For this review, take the finished solid that the model builds, in its own axes (mm). A direction names the side the tool comes from. Give positions to 0.01 mm unless a question says otherwise; leave off trailing zeros. Write each loop counter-clockwise with the first axis right and the second up, starting at its lowest first coordinate (ties: lowest second). Pieces come first, ordered by that corner, then holes. Notation, with made-up numbers: M 62.5,21 L 84.5,21 A34 cw 84.5,51 Z; hole C 35,13.5 d4. An arc over 180 degrees is marked long. One line per item, written item: value. Start each with the question number.
Item 1: Consider section B-B, the plane y = 35.5. Give the number of separate pieces and of enclosed holes in the cut face, and give its area (3 significant figures).
Item 2: Tool access review of faces 4 (the face through (-21.958, 49.233, 61.115)), 5 (the face through (-18.739, 41, 58)), 6 (the face through (-8.96, 43, 63)), 7 (the face through (53.62, 34.34, 48.98)): name each direction out of +Z, -Z, +X, -X, +Y, -Y from which nothing blocks a thin tool from reaching the whole face with its end or side.
Item 3: Consider section D-D, the plane y = 47. Write out the cut boundary in (x, z).
Item 4: Consider section C-C, the plane z = 41. Write out the cut boundary in (x, y).
Item 5: Clearance check with flat-ended pins moving along their axes: pin 1 Ø4 at (x, z) = (55.25, 77) entering from +Y; pin 2 Ø4 at (x, z) = (51, 32) entering from +Y; pin 3 Ø4 at (x, z) = (55.25, 49.05) entering from -Y. State where each tip first meets the part, or that it passes through.
Item 6: Mouldability with a two-part tool opening along Y and no side actions: class faces 1 (the face through (20, 47, 29.962)), 2 (the face through (-13.918, 52.936, 53.683)), 3 (the face through (57, 39.124, 78)) as released by +Y, released by -Y, zero draft, split by the parting line, or undercut.
Item 7: To check wall thickness, follow probe 1 along Z at (x, y) = (-13.5, 50.5); probe 2 along X at (y, z) = (51, 60.5); probe 3 along Z at (x, y) = (29.5, 51). State the ranges of each line that lie inside material, in increasing order.
Item 8: Consider section A-A, the plane x = -17.5. Write out the cut boundary in (y, z).
```python
from build123d import *

# Parameters (mm, degrees)
SKETCH2_W                                      = 90.675
SKETCH2_H                                      = 68.925
BOSS_EXTRUDE1_DEPTH                            = 6.35
SKETCH3_R                                      = 3.175
BOSS_EXTRUDE2_DEPTH                            = 4.7625
CSK_FOR_4_FLAT_HEAD_MACHINE_SCREW1_D           = 3.2639
CSK_FOR_4_FLAT_HEAD_MACHINE_SCREW1_CSINK_D     = 5.715
CSK_FOR_4_FLAT_HEAD_MACHINE_SCREW1_CSINK_ANGLE = 82
SKETCH10_W                                     = 90.675
SKETCH10_H                                     = 68.925
SKETCH10_W_2                                   = 77.975
SKETCH10_H_2                                   = 56.225
BOSS_EXTRUDE4_DEPTH                            = 25.4
SKETCH11_R                                     = 9.11225
SKETCH11_R_2                                   = 6.731
BOSS_EXTRUDE5_DEPTH                            = 9.779
CUT_EXTRUDE1_REACH                             = 144.676
SKETCH12_R                                     = 1.5875


with BuildPart() as part:
    # Sketch2 → Boss-Extrude1 (new body)
    with BuildSketch(Plane(origin=(0, 34.361183362, 0), x_dir=(-1, 0, 0), z_dir=(0, -1, 0))):
        with Locations((-20.248501783, -58.074565381)):
            Rectangle(SKETCH2_W, SKETCH2_H)
    extrude(amount=BOSS_EXTRUDE1_DEPTH)

    # Sketch3 → Boss-Extrude2 (add)
    with BuildSketch(Plane(origin=(0, 34.361183362, 0), x_dir=(-1, 0, 0), z_dir=(0, -1, 0))):
        with Locations(Location((-4.448501783, -33.899565381, 0), (0, 0, 90))):
            Circle(SKETCH3_R)
        with Locations(Location((-55.248501783, -49.049565381, 0), (0, 0, 90))):
            Circle(SKETCH3_R)
        with Locations(Location((-55.248501783, -76.999565381, 0), (0, 0, 90))):
            Circle(SKETCH3_R)
        with Locations(Location((-3.048501783, -82.199565381, 0), (0, 0, 90))):
            Circle(SKETCH3_R)
    extrude(amount=-BOSS_EXTRUDE2_DEPTH)

    # CSK for #4 Flat Head Machine Screw1 (through all)
    with Locations(Plane(origin=(0, 28.011183362, 0), x_dir=(-1, 0, 0), z_dir=(0, -1, 0))):
        with Locations((-3.048501783, -82.199565381), (-55.248501783, -76.999565381), (-55.248501783, -49.049565381), (-4.448501783, -33.899565381)):
            CounterSinkHole(CSK_FOR_4_FLAT_HEAD_MACHINE_SCREW1_D / 2, CSK_FOR_4_FLAT_HEAD_MACHINE_SCREW1_CSINK_D / 2, counter_sink_angle=CSK_FOR_4_FLAT_HEAD_MACHINE_SCREW1_CSINK_ANGLE)

    # Sketch10 → Boss-Extrude4 (add)
    with BuildSketch(Plane(origin=(0, 34.361183362, 0), x_dir=(1, 0, 0), z_dir=(0, 1, 0))):
        with Locations((20.248501783, -58.074565381)):
            Rectangle(SKETCH10_W, SKETCH10_H)
        with Locations((20.248501783, -58.074565381)):
            Rectangle(SKETCH10_W_2, SKETCH10_H_2, mode=Mode.SUBTRACT)
    extrude(amount=BOSS_EXTRUDE4_DEPTH)

    # Sketch11 → Boss-Extrude5 (add)
    with BuildSketch(Plane(origin=(-18.738998217, 0, 0), x_dir=(0, 0, -1), z_dir=(1, 0, 0))):
        with Locations((-62.374565381, 50.198683362)):
            Circle(SKETCH11_R)
        with Locations((-62.374565381, 50.198683362)):
            Circle(SKETCH11_R_2, mode=Mode.SUBTRACT)
    extrude(amount=BOSS_EXTRUDE5_DEPTH)

    # Sketch12 → Cut-Extrude1 (cut, up to next)
    with BuildSketch(Plane.ZY.offset(25.088998217), mode=Mode.PRIVATE) as cut_extrude1_sk1:
        with Locations((62.374565381, 50.198683362)):
            Circle(SKETCH12_R)
    cut_extrude1_tool1 = extrude(cut_extrude1_sk1.sketch, amount=-CUT_EXTRUDE1_REACH, mode=Mode.PRIVATE) & part.part
    add(cut_extrude1_tool1.solids().sort_by_distance((-25.088998, 50.198683, 62.374565))[0], mode=Mode.SUBTRACT)


solid = part.part
```
Model answer:
1. separate pieces: 5
1. enclosed holes: 5
1. area: 1,960 mm2
2. face 4: -X
2. face 5: none
2. face 6: +Y
2. face 7: +Y, -Y
3. outline: M -25.09,23.61 L 65.59,23.61 L 65.59,92.54 L -25.09,92.54 Z; hole M -18.74,29.96 L 59.24,29.96 L 59.24,86.19 L -18.74,86.19 L -18.74,70.91 L -8.96,70.91 L -8.96,68.3 L -18.74,68.3 L -18.74,56.45 L -8.96,56.45 L -8.96,53.84 L -18.74,53.84 Z
4. outline: M -25.09,28.01 L 65.59,28.01 L 65.59,59.76 L 59.24,59.76 L 59.24,34.36 L -18.74,34.36 L -18.74,59.76 L -25.09,59.76 Z
5. pin 1: stops at y = 39.12
5. pin 2: stops at y = 34.36
5. pin 3: stops at y = 29
6. face 1: zero draft
6. face 2: undercut
6. face 3: released by +Y
7. probe 1: z = 23.61 to 29.96, 53.27 to 55.65, 69.1 to 71.48, 86.19 to 92.54
7. probe 2: x = -25.09 to -18.74, 59.24 to 65.59
7. probe 3: z = 23.61 to 29.96, 86.19 to 92.54
8. outline: M 28.01,23.61 L 59.76,23.61 L 59.76,29.96 L 34.36,29.96 L 34.36,86.19 L 59.76,86.19 L 59.76,92.54 L 28.01,92.54 Z; C 50.2,62.37 d18.22; hole C 50.2,62.37 d13.46
